Geometry: final body of the model. Coordinates: model frame, mm. Give positions to 0.01 mm unless a question says otherwise; leave off trailing zeros. Write each loop counter-clockwise with the first axis right and the second up, starting at its lowest first coordinate (ties: lowest second). Pieces come first, ordered by that corner, then holes. Notation, with made-up numbers: M -18,43 L -4,43 A22 cw -4,69 Z; hole C 50,-12 d1. An arc over 180 degrees is marked long. Use a Markdown table: item, result. Add a question column.
(1) Cut plane B-B (x = -94). Output: boundary loops of the cut face in (y, z).
(2) Pin query (flat end, axial travel): pin 1 Ø3 at (y, z) = (-29, 2.5) entering from +X; pin 2 Ø1.8 at (y, z) = (-28, 2) entering from -X; pin 3 Ø1.8 at (x, z) = (-117.5, 4.5) entering from +Y. Return the tip coordinate at first contact, or that it passes through.
(3) Material intervals for L1, parallel to X at y = -23, z = 1.15; L2, parallel to Y at x = 93, z = 0.9; L3, parallel to X at y = -27, z = 4.8, sorted ascending.
(4) Cut plane A-A (y = -15). Output: boundary loops of the cut face in (x, z).
```python
from build123d import *

# Parameters (mm, degrees)
BOSS_EXTRUDE1_DEPTH = 6
CUT_EXTRUDE1_REACH  = 8
SKETCH2_W           = 20
SKETCH2_H           = 6
SKETCH2_W_2         = 6
CUT_EXTRUDE2_REACH  = 8
SKETCH3_W           = 17
SKETCH3_H           = 15.5


with BuildPart() as part:
    # Sketch1 → Boss-Extrude1 (new body)
    with BuildSketch(Plane.XY):
        Polygon((-85, -26.5), (-85, -32.5), (-35, -32.5), (-35, -26.5), (35, -26.5), (35, -32.5), (85, -32.5), (85, -26.5), (125, -26.5), (125, 32.5), (-125, 32.5), (-125, -26.5), align=None)
    extrude(amount=BOSS_EXTRUDE1_DEPTH)

    # Sketch2 → Cut-Extrude1 (cut, up to next)
    with BuildSketch(Plane.XY.offset(6), mode=Mode.PRIVATE) as cut_extrude1_sk1:
        with Locations((-80, 29.5)):
            Rectangle(SKETCH2_W, SKETCH2_H)
    cut_extrude1_tool1 = extrude(cut_extrude1_sk1.sketch, amount=-CUT_EXTRUDE1_REACH, mode=Mode.PRIVATE) & part.part
    add(cut_extrude1_tool1.solids().sort_by_distance((-80, 29.5, 6))[0], mode=Mode.SUBTRACT)
    # Sketch2 → Cut-Extrude1 (cut, up to next)
    with BuildSketch(Plane.XY.offset(6), mode=Mode.PRIVATE) as cut_extrude1_sk2:
        with Locations((-40, 29.5)):
            Rectangle(SKETCH2_W, SKETCH2_H)
    cut_extrude1_tool2 = extrude(cut_extrude1_sk2.sketch, amount=-CUT_EXTRUDE1_REACH, mode=Mode.PRIVATE) & part.part
    add(cut_extrude1_tool2.solids().sort_by_distance((-40, 29.5, 6))[0], mode=Mode.SUBTRACT)
    # Sketch2 → Cut-Extrude1 (cut, up to next)
    with BuildSketch(Plane.XY.offset(6), mode=Mode.PRIVATE) as cut_extrude1_sk3:
        with Locations((0, 29.5)):
            Rectangle(SKETCH2_W, SKETCH2_H)
    cut_extrude1_tool3 = extrude(cut_extrude1_sk3.sketch, amount=-CUT_EXTRUDE1_REACH, mode=Mode.PRIVATE) & part.part
    add(cut_extrude1_tool3.solids().sort_by_distance((0, 29.5, 6))[0], mode=Mode.SUBTRACT)
    # Sketch2 → Cut-Extrude1 (cut, up to next)
    with BuildSketch(Plane.XY.offset(6), mode=Mode.PRIVATE) as cut_extrude1_sk4:
        with Locations((40, 29.5)):
            Rectangle(SKETCH2_W, SKETCH2_H)
    cut_extrude1_tool4 = extrude(cut_extrude1_sk4.sketch, amount=-CUT_EXTRUDE1_REACH, mode=Mode.PRIVATE) & part.part
    add(cut_extrude1_tool4.solids().sort_by_distance((40, 29.5, 6))[0], mode=Mode.SUBTRACT)
    # Sketch2 → Cut-Extrude1 (cut, up to next)
    with BuildSketch(Plane.XY.offset(6), mode=Mode.PRIVATE) as cut_extrude1_sk5:
        with Locations((80, 29.5)):
            Rectangle(SKETCH2_W, SKETCH2_H)
    cut_extrude1_tool5 = extrude(cut_extrude1_sk5.sketch, amount=-CUT_EXTRUDE1_REACH, mode=Mode.PRIVATE) & part.part
    add(cut_extrude1_tool5.solids().sort_by_distance((80, 29.5, 6))[0], mode=Mode.SUBTRACT)
    # Sketch2 → Cut-Extrude1 (cut, up to next)
    with BuildSketch(Plane.XY.offset(6), mode=Mode.PRIVATE) as cut_extrude1_sk6:
        with Locations((-117, 29.5)):
            Rectangle(SKETCH2_W_2, SKETCH2_H)
    cut_extrude1_tool6 = extrude(cut_extrude1_sk6.sketch, amount=-CUT_EXTRUDE1_REACH, mode=Mode.PRIVATE) & part.part
    add(cut_extrude1_tool6.solids().sort_by_distance((-117, 29.5, 6))[0], mode=Mode.SUBTRACT)
    # Sketch2 → Cut-Extrude1 (cut, up to next)
    with BuildSketch(Plane.XY.offset(6), mode=Mode.PRIVATE) as cut_extrude1_sk7:
        with Locations((117, 29.5)):
            Rectangle(SKETCH2_W_2, SKETCH2_H)
    cut_extrude1_tool7 = extrude(cut_extrude1_sk7.sketch, amount=-CUT_EXTRUDE1_REACH, mode=Mode.PRIVATE) & part.part
    add(cut_extrude1_tool7.solids().sort_by_distance((117, 29.5, 6))[0], mode=Mode.SUBTRACT)

    # Sketch3 → Cut-Extrude2 (cut, up to next)
    with BuildSketch(Plane(origin=(0, 0, 0), x_dir=(-1, 0, 0), z_dir=(0, 0, -1)), mode=Mode.PRIVATE) as cut_extrude2_sk1:
        with Locations((-11.006971283, -19.65)):
            Rectangle(SKETCH3_W, SKETCH3_H)
    cut_extrude2_tool1 = extrude(cut_extrude2_sk1.sketch, amount=-CUT_EXTRUDE2_REACH, mode=Mode.PRIVATE) & part.part
    add(cut_extrude2_tool1.solids().sort_by_distance((11.006971, -19.65, 0))[0], mode=Mode.SUBTRACT)


solid = part.part
```
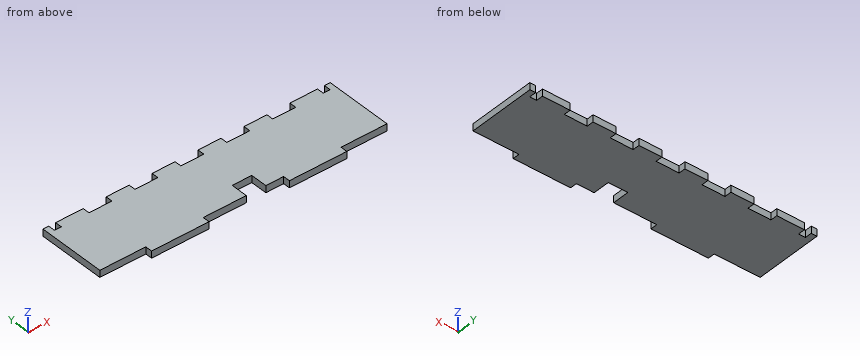
Answer list:
| question | item | result |
|---|---|---|
| 1 | outline | M -26.5,0 L 32.5,0 L 32.5,6 L -26.5,6 Z |
| 2 | pin 1 | x = 85 |
| 2 | pin 2 | x = -85 |
| 2 | pin 3 | y = 26.5 |
| 3 | L1 | -125 to 2.51, 19.51 to 125 |
| 3 | L2 | -26.5 to 32.5 |
| 3 | L3 | -85 to -35, 35 to 85 |
| 4 | outline | M -125,0 L 2.51,0 L 2.51,6 L -125,6 Z; M 19.51,0 L 125,0 L 125,6 L 19.51,6 Z |
